Could you check a few things on this model? Use its own coordinates, in mm. A direction names the side the tool comes from. Give positions to 0.01 mm unless a question says otherwise; leave off trailing zeros. Order: outer loops, then holes, each group sorted by start corner. A loop starts at its lowest first (then second) coordinate and runs counter-clockwise, first axis right, second up.
from build123d import *

# Parameters (mm, degrees)
BOSS_EXTRUDE1_DEPTH = 8
SKETCH2_R           = 2
CUT_EXTRUDE1_DEPTH  = 9
SKETCH3_R           = 2
SKETCH3_R_2         = 1.6
CUT_EXTRUDE2_DEPTH  = 9
SKETCH4_R           = 2.05
CUT_EXTRUDE3_DEPTH  = 6
SKETCH5_W           = 5
SKETCH5_H           = 10
BOSS_EXTRUDE2_DEPTH = 8
SKETCH6_R           = 1.55
CUT_EXTRUDE4_DEPTH  = 128.5


with BuildPart() as part:
    # Sketch1 → Boss-Extrude1 (new body)
    with BuildSketch(Plane(origin=(0, 0, 0), x_dir=(1, 0, 0), z_dir=(0, 1, 0))):
        Polygon((70, 34), (-62, 34), (-62, 7.645012604), (-65, 7.645012604), (-65, -16.427077226), (-70, -21.427077226), (-70, -31), (-65, -31), (-62, -34), (8, -34), (8, -39), (14, -39), (14, -34), (42, -34), (42, -39), (48, -39), (48, -34), (62, -34), (65, -31), (70, -31), (70, -23.155364425), (67, -20.155364425), (67, -0.506394588), (70, -0.506394588), align=None)
    extrude(amount=BOSS_EXTRUDE1_DEPTH)

    # Sketch2 → Cut-Extrude1 (cut, through all)
    with BuildSketch(Plane(origin=(0, 8, 0), x_dir=(1, 0, 0), z_dir=(0, 1, 0))):
        with Locations((0, 8)):
            Circle(SKETCH2_R)
        with Locations((0, -8)):
            Circle(SKETCH2_R)
    extrude(amount=-CUT_EXTRUDE1_DEPTH, mode=Mode.SUBTRACT)

    # Sketch3 → Cut-Extrude2 (cut, through all)
    with BuildSketch(Plane(origin=(0, 8, 0), x_dir=(1, 0, 0), z_dir=(0, 1, 0))):
        with Locations((57, -7)):
            Circle(SKETCH3_R)
        with Locations((-37, 22)):
            Circle(SKETCH3_R_2)
        with Locations((-27, 22)):
            Circle(SKETCH3_R_2)
        with Locations((30, 22)):
            Circle(SKETCH3_R_2)
        with Locations((40, 22)):
            Circle(SKETCH3_R_2)
        with Locations((-55, -7)):
            Circle(SKETCH3_R)
    extrude(amount=-CUT_EXTRUDE2_DEPTH, mode=Mode.SUBTRACT)

    # Sketch4 → Cut-Extrude3 (cut)
    with BuildSketch(Plane(origin=(67, 0, 0), x_dir=(0, 0, -1), z_dir=(1, 0, 0))):
        with Locations((-6.506394588, 4)):
            Circle(SKETCH4_R)
    extrude(amount=-CUT_EXTRUDE3_DEPTH, mode=Mode.SUBTRACT)

    # Sketch5 → Boss-Extrude2 (add)
    with BuildSketch(Plane(origin=(0, 8, 0), x_dir=(1, 0, 0), z_dir=(0, 1, 0))):
        with Locations((-55, -19)):
            Rectangle(SKETCH5_W, SKETCH5_H)
        with Locations((-55, 22)):
            Rectangle(SKETCH5_W, SKETCH5_H)
        with Locations((57, -19)):
            Rectangle(SKETCH5_W, SKETCH5_H)
        with Locations((62, 22)):
            Rectangle(SKETCH5_W, SKETCH5_H)
    extrude(amount=BOSS_EXTRUDE2_DEPTH)

    # Sketch6 → Cut-Extrude4 (cut, through all)
    with BuildSketch(Plane.ZY.offset(57.5)):
        with Locations((-22, 12)):
            Circle(SKETCH6_R)
        with Locations((19, 12)):
            Circle(SKETCH6_R)
    extrude(amount=-CUT_EXTRUDE4_DEPTH, mode=Mode.SUBTRACT)


solid = part.part
Item 1: For faces 1 (the flat face through (67, 4, 31)), 2 (the flat face through (-55, 12, -17)), 3 (the flat face through (28, 4, 34)), which set-ups out of +Z, -Z, +X, -X, +Y, -Y let a thin tool reach every point of the face, with its end or its side?
Findings:
face 1: +Z, +X, +Y, -Y
face 2: +X, -X, +Y
face 3: +Z, +Y, -Y
Item 2: Imagine slicing it at C-C on z = -25. List the corners of the cut face in (x, y) for me.
Findings:
outline: (-62, 0) - (70, 0) - (70, 8) - (64.5, 8) - (64.5, 16) - (59.5, 16) - (59.5, 8) - (-52.5, 8) - (-52.5, 16) - (-57.5, 16) - (-57.5, 8) - (-62, 8) - close
Item 3: Please list where these lines run through material, in increasing order: line 1 along X through (y, z) = (2.75, -22); line 2 along Z through (x, y) = (-55, 5); line 3 along Z through (x, y) = (-27, 6.75).
Findings:
line 1: x = -62 to -38.6, -35.4 to -28.6, -25.4 to 28.4, 31.6 to 38.4, 41.6 to 70
line 2: z = -34 to 5, 9 to 34
line 3: z = -34 to -23.6, -20.4 to 34
Item 4: Imagine slicing it at B-B on x = -37. List the corners of the cut face in (y, z) for me.
Findings:
outline: (0, -34) - (8, -34) - (8, -23.6) - (0, -23.6) - close; (0, -20.4) - (8, -20.4) - (8, 34) - (0, 34) - close
Item 5: Imagine slicing it at A-A on x = 57. List the corners of the cut face in (y, z) for me.
Findings:
outline: (0, -34) - (8, -34) - (8, 5) - (0, 5) - close; (0, 9) - (8, 9) - (8, 14) - (16, 14) - (16, 24) - (8, 24) - (8, 34) - (0, 34) - close; hole circle Ø3.1 at (12, 19)
Item 6: We'd pull the mould along Z, two halves only. Please class faces 4 (the cylindrical face through (-28.18, 4.06, -23.08)), 5 (the flat face through (-55, 12, -27)), 6 (the flat face through (-55, 16, -22)): +Z half, -Z half, draft (parallel to the pull), parting line (faces both ways), or undercut.
Findings:
face 4: undercut
face 5: -Z half
face 6: draft
Item 7: For pin 1 (1.9 mm diameter, centred on y = 12, z = -22, fed in from +X); pin 2 (4 mm diameter, centred on y = 12.5, z = 17, fed in from +X); pin 3 (6 mm diameter, centred on x = -50, y = 12, fed in from -Z); pin 4 (1.5 mm diameter, centred on x = 67, y = 5.5, fed in from +Z), each with a flat end and sliding along its axis, tell me the tip position at first contact or that it passes through.
Findings:
pin 1: passes through
pin 2: stops at x = 59.5
pin 3: stops at z = -27
pin 4: stops at z = 31
Item 8: Imagine slicing it at D-D on z = 27. List the corners of the cut face in (x, y) for me, then the cut area to 3 significant figures.
Findings:
outline: (-70, 0) - (70, 0) - (70, 8) - (-70, 8) - close
area: 1,120 mm2
